from build123d import *

# Parameters (mm, degrees)
SKETCH_1_R                = 47
EXTRUDE_1_DEPTH           = 40
CUT_EXTRUDE_1_DEPTH       = 78.575769413
CUT_EXTRUDE_1_DEPTH_BACK  = 78.575769413
FILLET_1_R                = 3
HOLE_WIZARD_1_D           = 3.6
HOLE_WIZARD_1_CBORE_D     = 6
HOLE_WIZARD_1_CBORE_DEPTH = 3.4
PATTERN_CIRCULAR_1_COUNT  = 4
SHELL_START               = 3
SHELL_1_DEPTH             = 35.812510714
SHELL_START_2             = 6.4
SHELL_1_2_DEPTH           = 32.412510714


# Read off the part's stored shape, not the designer's step: 抽壳1
with BuildPart() as part:
    # 草图1 → 凸台-拉伸1 (new body)
    with BuildSketch(Plane.XY):
        Circle(SKETCH_1_R)
    extrude(amount=EXTRUDE_1_DEPTH)

    # 草图2 → 切除-拉伸1 (cut, two sides: drawn at the far end of the back side and taken through both)
    with BuildSketch(Plane(origin=(0, 0, 0), x_dir=(0, 0, -1), z_dir=(1, 0, 0)).offset(-CUT_EXTRUDE_1_DEPTH_BACK)):
        Polygon((-40, 47), (-40, -47), (-5.786797979, -47), align=None)
    extrude(amount=CUT_EXTRUDE_1_DEPTH + CUT_EXTRUDE_1_DEPTH_BACK, mode=Mode.SUBTRACT)

    # 圆角1
    fillet_1_edges = [part.edges().sort_by_distance(p)[0] for p in [
        (-47, 0, 0),
    ]]
    fillet(fillet_1_edges, radius=FILLET_1_R)

    # 打孔尺寸(%根据)内六角圆柱头螺钉的类型1 (through all)
    with Locations(Plane(origin=(0, 0, 0), x_dir=(-1, 0, 0), z_dir=(0, 0, -1))):
        with Locations((0, 43.75)):
            hole_wizard_1 = CounterBoreHole(HOLE_WIZARD_1_D / 2, HOLE_WIZARD_1_CBORE_D / 2, HOLE_WIZARD_1_CBORE_DEPTH)

    # 阵列(圆周)1: 打孔尺寸(%根据)内六角圆柱头螺钉的类型1 ×4 about axis
    pattern_circular_1_axis = Axis((0, 0, 0), (0, 0, 1))
    for i in range(1, PATTERN_CIRCULAR_1_COUNT):
        add(hole_wizard_1.rotate(pattern_circular_1_axis, i * 360 / PATTERN_CIRCULAR_1_COUNT), mode=Mode.SUBTRACT)

    # 抽壳1 outline → 抽壳1 (cut)
    with BuildSketch(Plane.XY.offset(SHELL_START)):
        with BuildLine():
            ThreePointArc((-43.589285714, -5.99784719), (-31.112698372, -31.112698372), (-5.99784719, -43.589285714))
            ThreePointArc((-5.99784719, -43.589285714), (0, -37.75), (5.99784719, -43.589285714))
            ThreePointArc((5.99784719, -43.589285714), (31.112698372, -31.112698372), (43.589285714, -5.99784719))
            ThreePointArc((43.589285714, -5.99784719), (37.75, 0), (43.589285714, 5.99784719))
            ThreePointArc((43.589285714, 5.99784719), (31.112698372, 31.112698372), (5.99784719, 43.589285714))
            ThreePointArc((5.99784719, 43.589285714), (0, 37.75), (-5.99784719, 43.589285714))
            ThreePointArc((-5.99784719, 43.589285714), (-31.112698372, 31.112698372), (-43.589285714, 5.99784719))
            ThreePointArc((-43.589285714, 5.99784719), (-37.75, 0), (-43.589285714, -5.99784719))
        make_face()
    extrude(amount=SHELL_1_DEPTH, mode=Mode.SUBTRACT)

    # Shell 1 2 outline → Shell 1 2 (cut)
    with BuildSketch(Plane.XY.offset(SHELL_START_2)):
        with BuildLine():
            ThreePointArc((5.99784719, -43.589285714), (0, -37.75), (-5.99784719, -43.589285714))
            ThreePointArc((-5.99784719, -43.589285714), (-5.399423225, -43.66745045), (-4.799983462, -43.7374))
            ThreePointArc((-4.799983462, -43.7374), (0, -38.95), (4.799983462, -43.7374))
            ThreePointArc((4.799983462, -43.7374), (5.399423225, -43.66745045), (5.99784719, -43.589285714))
        make_face()
        with BuildLine():
            ThreePointArc((-43.7374, -4.799983462), (-43.66745045, -5.399423225), (-43.589285714, -5.99784719))
            ThreePointArc((-43.589285714, -5.99784719), (-37.75, 0), (-43.589285714, 5.99784719))
            ThreePointArc((-43.589285714, 5.99784719), (-43.66745045, 5.399423225), (-43.7374, 4.799983462))
            ThreePointArc((-43.7374, 4.799983462), (-38.95, 0), (-43.7374, -4.799983462))
        make_face()
        with BuildLine():
            ThreePointArc((43.589285714, 5.99784719), (37.75, 0), (43.589285714, -5.99784719))
            ThreePointArc((43.589285714, -5.99784719), (43.66745045, -5.399423225), (43.7374, -4.799983462))
            ThreePointArc((43.7374, -4.799983462), (38.95, 0), (43.7374, 4.799983462))
            ThreePointArc((43.7374, 4.799983462), (43.66745045, 5.399423225), (43.589285714, 5.99784719))
        make_face()
        with BuildLine():
            ThreePointArc((-4.799983462, 43.7374), (-5.399423225, 43.66745045), (-5.99784719, 43.589285714))
            ThreePointArc((-5.99784719, 43.589285714), (0, 37.75), (5.99784719, 43.589285714))
            ThreePointArc((5.99784719, 43.589285714), (5.399423225, 43.66745045), (4.799983462, 43.7374))
            ThreePointArc((4.799983462, 43.7374), (0, 38.95), (-4.799983462, 43.7374))
        make_face()
    extrude(amount=SHELL_1_2_DEPTH, mode=Mode.SUBTRACT)


solid = part.part
Input: part model. Units: mm. Frame: model coordinates. A direction names the side the tool comes from. Coordinates: 2 decimals unless noted, no trailing zeros. Loops run counter-clockwise (first coordinate to the right, second up) from the corner with the lowest first, then second, coordinate; pieces in that order, holes last.
(1) Material intervals for probe 1 along X at (y, z) = (1.5, 14); probe 2 along Z at (x, y) = (7, 21.5); probe 3 along X at (y, z) = (0, 1.05), sorted ascending.
(2) Pull-direction query (Y, two-part tool) for faces 1 (the face through (41.558, -0.219, 22.814)), 2 (the face through (-6.12, 46.6, 17.13)), 3 (the face through (-38.95, 0.11, 15.39)); classes: released by +Y, released by -Y, zero draft, split by the parting line, or undercut.
(3) Section D-D on z = 16. Return the cut outline in (x, y).
(4) Section B-B on x = 0. Return the cut outline in (y, z), then the cut area to 3 significant figures.
(5) First-contact query: pin 1 Ø2 at (y, z) = (24.5, 24.5) entering from -X; pin 2 Ø4.5 at (x, y) = (-43.75, 0) entering from +Z; pin 3 Ø8 at (y, z) = (14.5, 28.5) entering from +X. Flat tips, straight axial feed; report the tip coordinate or a pass-through.
(6) Section C-C on z = 28.5. Return the cut outline in (x, y), then the cut area to 3 significant figures.
(7) Set-up query: faces 4 (the face through (-44.291, 1.717, 13.615)), 5 (the face through (42, 1, 3.4)), 6 (the face through (0.4, -38.7, 6.4)). Return all of +Z, -Z, +X, -X, +Y, -Y with unobstructed straight access to the full face (end or side cutting, diameter ignored); none if empty.
(8) Section A-A on y = 0. Return the cut outline in (x, z).
Data:
1. probe 1: x = -46.98 to -44.74, -42.76 to -39.19, 39.19 to 42.76, 44.74 to 46.98
1. probe 2: z = 0 to 3
1. probe 3: x = -40.75 to 40.75
2. face 1: released by -Y
2. face 2: split by the parting line
2. face 3: undercut
3. outline: (-43.74, -4.8) arc R4.8 ccw to (-43.74, 4.8) arc R44 cw to (-43.59, 6) arc R44 cw to (-6, 43.59) arc R44 cw to (-4.8, 43.74) arc R4.8 ccw to (4.8, 43.74) arc R44 cw to (6, 43.59) arc R44 cw to (43.59, 6) arc R44 cw to (43.74, 4.8) arc R4.8 ccw to (43.74, -4.8) arc R44 cw to (43.59, -6) arc R44 cw to (39.72, -18.94) - (43.02, -18.94) arc R47 ccw (long way) to (-43.02, -18.94) - (-39.72, -18.94) arc R44 cw to (-43.59, -6) arc R44 cw to start; hole circle Ø3.6 at (-43.75, 0); hole circle Ø3.6 at (0, 43.75); hole circle Ø3.6 at (43.75, 0)
4. outline: (-47, 3) arc R3 ccw to (-46.75, 1.8) - (-46.75, 3.4) - (-45.55, 3.4) - (-45.55, 6.31) - (-47, 5.79) - close; (-41.95, 3.4) - (-40.75, 3.4) - (-40.75, 0) - (40.75, 0) - (40.75, 3.4) - (41.95, 3.4) - (41.95, 38.16) - (38.95, 37.07) - (38.95, 6.4) - (37.75, 6.4) - (37.75, 3) - (-37.75, 3) - (-37.75, 6.4) - (-38.95, 6.4) - (-38.95, 8.72) - (-41.95, 7.62) - close; (45.55, 3.4) - (46.75, 3.4) - (46.75, 1.8) arc R3 ccw to (47, 3) - (47, 40) - (45.55, 39.47) - close
4. area: 428 mm2
5. pin 1: stops at x = -40.7
5. pin 2: stops at z = 23.71
5. pin 3: stops at x = 45.73
6. outline: (-44.4, 15.4) - (-41.22, 15.4) arc R44 cw to (-6, 43.59) arc R44 cw to (-4.8, 43.74) arc R4.8 ccw to (4.8, 43.74) arc R44 cw to (6, 43.59) arc R44 cw to (41.22, 15.4) - (44.4, 15.4) arc R47 ccw to start; hole circle Ø3.6 at (0, 43.75)
6. area: 362 mm2
7. face 4: +Z, -Z
7. face 5: -Z
7. face 6: +Z
8. outline: (-47, 3) arc R3 ccw to (-46.75, 1.8) - (-46.75, 3.4) - (-45.55, 3.4) - (-45.55, 22.89) - (-47, 22.89) - close; (-41.95, 3.4) - (-40.75, 3.4) - (-40.75, 0) - (40.75, 0) - (40.75, 3.4) - (41.95, 3.4) - (41.95, 22.89) - (38.95, 22.89) - (38.95, 6.4) - (37.75, 6.4) - (37.75, 3) - (-37.75, 3) - (-37.75, 6.4) - (-38.95, 6.4) - (-38.95, 22.89) - (-41.95, 22.89) - close; (45.55, 3.4) - (46.75, 3.4) - (46.75, 1.8) arc R3 ccw to (47, 3) - (47, 22.89) - (45.55, 22.89) - close
